Could you check a few things on this model? Use its own coordinates, in mm. Face numbers are marked on the shaded views. A direction names the side the tool comes from. Coordinates: 2 decimals unless noted, no trailing zeros. Order: outer loops, then holes, each group sorted by start corner. A loop starts at its lowest first (then second) coordinate and runs counter-clockwise, first axis right, second up. Notation, with made-up numbers: (60, 4) - (75, 4) arc R17 ccw to (75, 12) - close; hole circle Ø3 at (71, -28). An arc over 180 degrees is marked (long way). One line per item, written item: value.
from build123d import *

# Parameters (mm, degrees)
SKETCH1_W                = 20
SKETCH1_H                = 20
SKETCH1_R                = 5
BOSS_EXTRUDE1_DEPTH      = 5
SKETCH2_W                = 5
SKETCH2_H                = 20
BOSS_EXTRUDE2_DEPTH      = 20
BOSS_EXTRUDE6_DEPTH      = 20
BOSS_EXTRUDE7_DEPTH      = 40
BOSS_EXTRUDE7_DEPTH_BACK = 60
SKETCH9_W                = 75
SKETCH9_H                = 10


with BuildPart() as part:
    # Sketch1 → Boss-Extrude1 (new body)
    with BuildSketch(Plane.XY):
        Rectangle(SKETCH1_W, SKETCH1_H)
        Circle(SKETCH1_R, mode=Mode.SUBTRACT)
    extrude(amount=BOSS_EXTRUDE1_DEPTH)

    # Sketch2 → Boss-Extrude2 (add)
    with BuildSketch(Plane.ZY.offset(10)):
        with Locations((2.5, 0)):
            Rectangle(SKETCH2_W, SKETCH2_H)
    extrude(amount=BOSS_EXTRUDE2_DEPTH)

    # Sketch8 → Boss-Extrude6 (add)
    with BuildSketch(Plane.XZ.offset(10)):
        Polygon((35.075402168, 114.183233441), (-39.924597832, 114.183233441), (-34.924597832, 110.86660865), (-39.357847412, 104.183233441), (35.075402168, 104.183233441), align=None)
        Polygon((-34.924597832, 110.86660865), (-39.924597832, 114.183233441), (-39.924597832, 104.183233441), (-39.357847412, 104.183233441), align=None)
        Polygon((-39.924597832, 114.183233441), (-66.457596155, 74.183233441), (-60.457596155, 74.183233441), (-60.457596155, 72.374165373), (-39.357847412, 104.183233441), (-39.924597832, 104.183233441), align=None)
        Polygon((-60.457596155, 74.183233441), (-66.457596155, 74.183233441), (-61.457596155, 70.86660865), (-60.457596155, 72.374165373), align=None)
        Polygon((-66.457596155, 74.183233441), (-66.457596155, 24.183233441), (-63.140971364, 29.183233441), (-60.457596155, 27.403283692), (-60.457596155, 72.374165373), (-61.457596155, 70.86660865), align=None)
        Polygon((-63.140971364, 29.183233441), (-66.457596155, 24.183233441), (-60.457596155, 24.183233441), (-60.457596155, 27.403283692), align=None)
        Polygon((-66.457596155, 24.183233441), (-30, 0), (-30, 5), (-26.68337521, 5), (-60.457596155, 27.403283692), (-60.457596155, 24.183233441), align=None)
    extrude(amount=-BOSS_EXTRUDE6_DEPTH)

    # Sketch9 → Boss-Extrude7 (add, two sides: drawn at the far end of the back side and taken through both)
    with BuildSketch(Plane.XZ.offset(10).offset(-BOSS_EXTRUDE7_DEPTH_BACK)):
        with Locations((-2.424597832, 109.183233441)):
            Rectangle(SKETCH9_W, SKETCH9_H)
    extrude(amount=BOSS_EXTRUDE7_DEPTH + BOSS_EXTRUDE7_DEPTH_BACK)


solid = part.part
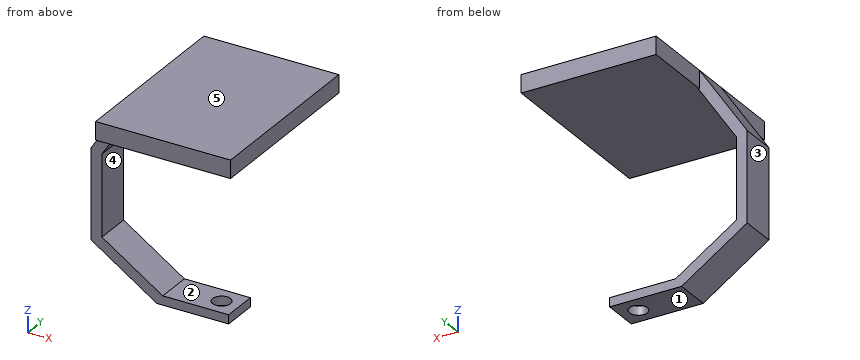
Item 1: I want a section at B-B on y = 0. Please give me the cut outline in (x, z).
Conclusion:
outline: (-66.46, 24.18) - (-30, 0) - (-5, 0) - (-5, 5) - (-26.68, 5) - (-60.46, 27.4) - (-60.46, 72.37) - (-39.36, 104.18) - (35.08, 104.18) - (35.08, 114.18) - (-39.92, 114.18) - (-66.46, 74.18) - close; (5, 0) - (10, 0) - (10, 5) - (5, 5) - close
Item 2: If I drill on probe 1 along Y at (x, z) = (0, 2); probe 2 along Z at (x, y) = (-5.5, 0.5); probe 3 along Z at (x, y) = (-22.5, 28), over which ranges is the centre line in solid material (lowest first)?
Conclusion:
probe 1: -10 to -5, 5 to 10
probe 2: 0 to 5, 104.18 to 114.18
probe 3: 104.18 to 114.18
Item 3: I'm going to push flat-ended pins straight in: pin 1 Ø6 at (x, y) = (-40, 8.5) entering from +Z; pin 2 Ø3 at (y, z) = (-37.5, 107) entering from -X; pin 3 Ø3 at (y, z) = (2.5, 62.5) entering from +X; pin 4 Ø2.5 at (y, z) = (0.5, 2) entering from +X. Where does each tip first touch, or does it pass through?
Conclusion:
pin 1: z = 114.18
pin 2: x = -39.92
pin 3: x = -60.46
pin 4: x = 10
Item 4: I want a section at D-D on z = 40. Please give me the cut outline in (x, y).
Conclusion:
outline: (-66.46, -10) - (-60.46, -10) - (-60.46, 10) - (-66.46, 10) - close
Item 5: I want a section at A-A on x = -22.5. Please give me the cut outline in (y, z).
Conclusion:
outline: (-50, 104.18) - (50, 104.18) - (50, 114.18) - (-50, 114.18) - close; (-10, 0) - (10, 0) - (10, 5) - (-10, 5) - close
Item 6: Thinking about a two-plate mould opening in Z: for the marked faces 1, 2 and 3, which applies, pulls with the +Z half, pulls with the -Z half, needs draft (parallel to the pull), parting line crosses it, or undercut?
Conclusion:
face 1: pulls with the -Z half
face 2: undercut
face 3: needs draft
Item 7: I want a section at C-C on x = 0. Please give me the cut outline in (y, z), then the cut area to 3 significant figures.
Conclusion:
outline: (-50, 104.18) - (50, 104.18) - (50, 114.18) - (-50, 114.18) - close; (-10, 0) - (-5, 0) - (-5, 5) - (-10, 5) - close; (5, 0) - (10, 0) - (10, 5) - (5, 5) - close
area: 1,050 mm²
Item 8: For the marked faces 4 and 5, which set-ups out of +Z, -Z, +X, -X, +Y, -Y let a thin tool reach every point of the face, with its end or its side?
Conclusion:
face 4: +X, +Y, -Y
face 5: +Z, +X, -X, +Y, -Y
